from build123d import *

# Parameters (mm, degrees)
CROQUIS1_W              = 36
CROQUIS1_H              = 36
SALIENTE_EXTRUIR1_DEPTH = 13
CROQUIS5_R              = 1.5
CORTAR_EXTRUIR2_DEPTH   = 13
CROQUIS6_W              = 36
CROQUIS6_H              = 36
CROQUIS6_R              = 2.5
CORTAR_EXTRUIR3_DEPTH   = 5
CROQUIS7_W              = 36
CROQUIS7_H              = 36
CROQUIS7_R              = 2.7
CORTAR_EXTRUIR4_DEPTH   = 5
CROQUIS8_W              = 9
CROQUIS8_H              = 10
CROQUIS8_W_2            = 11
CORTAR_EXTRUIR5_DEPTH   = 3


with BuildPart() as part:
    # Croquis1 → Saliente-Extruir1 (new body)
    with BuildSketch(Plane.XY):
        with Locations((-24.893753741, 2.264150943)):
            Rectangle(CROQUIS1_W, CROQUIS1_H)
    extrude(amount=SALIENTE_EXTRUIR1_DEPTH)

    # Croquis5 → Cortar-Extruir2 (cut)
    with BuildSketch(Plane(origin=(0, 0, 0), x_dir=(-1, 0, 0), z_dir=(0, 0, -1))):
        with Locations((40.143753741, 17.514150943)):
            Circle(CROQUIS5_R)
        with Locations((40.143753741, -12.985849057)):
            Circle(CROQUIS5_R)
        with Locations((9.643753741, -12.985849057)):
            Circle(CROQUIS5_R)
        with Locations((9.643753741, 17.514150943)):
            Circle(CROQUIS5_R)
    extrude(amount=-CORTAR_EXTRUIR2_DEPTH, mode=Mode.SUBTRACT)

    # Croquis6 → Cortar-Extruir3 (cut)
    with BuildSketch(Plane(origin=(0, 0, 0), x_dir=(-1, 0, 0), z_dir=(0, 0, -1))):
        with Locations((24.893753741, 2.264150943)):
            Rectangle(CROQUIS6_W, CROQUIS6_H)
        with Locations((40.143753741, 17.514150943)):
            Circle(CROQUIS6_R, mode=Mode.SUBTRACT)
        with Locations((9.643753741, 17.514150943)):
            Circle(CROQUIS6_R, mode=Mode.SUBTRACT)
        with Locations((40.143753741, -12.985849057)):
            Circle(CROQUIS6_R, mode=Mode.SUBTRACT)
        with Locations((9.643753741, -12.985849057)):
            Circle(CROQUIS6_R, mode=Mode.SUBTRACT)
    extrude(amount=-CORTAR_EXTRUIR3_DEPTH, mode=Mode.SUBTRACT)

    # Croquis7 → Cortar-Extruir4 (cut)
    with BuildSketch(Plane.XY.offset(13)):
        with Locations((-24.893753741, 2.264150943)):
            Rectangle(CROQUIS7_W, CROQUIS7_H)
        with Locations((-40.143753741, 17.514150943)):
            Circle(CROQUIS7_R, mode=Mode.SUBTRACT)
        with Locations((-9.643753741, 17.514150943)):
            Circle(CROQUIS7_R, mode=Mode.SUBTRACT)
        with Locations((-40.143753741, -12.985849057)):
            Circle(CROQUIS7_R, mode=Mode.SUBTRACT)
        with Locations((-9.643753741, -12.985849057)):
            Circle(CROQUIS7_R, mode=Mode.SUBTRACT)
    extrude(amount=-CORTAR_EXTRUIR4_DEPTH, mode=Mode.SUBTRACT)

    # Croquis8 → Cortar-Extruir5 (cut)
    with BuildSketch(Plane.XY.offset(8)):
        with Locations((-32.393753741, -4.735849057)):
            Rectangle(CROQUIS8_W, CROQUIS8_H)
        with Locations((-32.393753741, 9.264150943)):
            Rectangle(CROQUIS8_W, CROQUIS8_H)
        with Locations((-18.393753741, -4.735849057)):
            Rectangle(CROQUIS8_W_2, CROQUIS8_H)
        with Locations((-18.393753741, 9.264150943)):
            Rectangle(CROQUIS8_W_2, CROQUIS8_H)
    extrude(amount=-CORTAR_EXTRUIR5_DEPTH, mode=Mode.SUBTRACT)


solid = part.part
Here's how the part is built. I have some questions about the finished solid (model axes, mm). A direction names the side the tool comes from. Coordinates: 2 decimals unless noted, no trailing zeros. Order: outer loops, then holes, each group sorted by start corner. A loop starts at its lowest first (then second) coordinate and runs counter-clockwise, first axis right, second up. Notation, with made-up numbers: M 35.5,38.25 L 93.5,38.25 A28 ccw 93.5,68.25 Z; hole C 84,37.5 d10. An arc over 180 degrees is marked long. Answer as CSV lines item,"result". Start each with the question number.
1. For pin 1 (1.5 mm diameter, centred on y = -10, z = 1.5, fed in from +X); pin 2 (2 mm diameter, centred on x = -35, y = -9, fed in from +Z); pin 3 (18 mm diameter, centred on x = -33.5, y = -4, fed in from -Z), each with a flat end and sliding along its axis, tell me the tip position at first contact or that it passes through.
2. I want a section at A-A, the plane z = 11. Write out the boundary of the cut face in (x, y), and give its area (3 significant figures).
3. I want a section at C-C, the plane y = -8. Write out the boundary of the cut face in (x, z), and give its area (3 significant figures).
4. I need wall thicknesses on line 1 (X direction, y = 7.5, z = 5.25); line 2 (X direction, y = 17.5, z = 3.25); line 3 (X direction, y = 17, z = 5.5). Which ranges of each line are inside material? Lowest first, please. Write a range as [from, to].
5. I want a section at B-B, the plane x = -19. Write out the boundary of the cut face in (y, z).
6. I want a section at D-D, the plane z = 2.5. Write out the boundary of the cut face in (x, y).
7. On a 3-axis mill with a long thin cutter (end or side, diameter ignored), from which of +Z, -Z, +X, -X, +Y, -Y can I reach the whole of each face in a straight line? I mean faces 1 (the cylindrical face through (-9.318, 19.993, 2.465)), 2 (the cylindrical face through (-42.134, 19.339, 10.535)), 3 (the flat face through (-6.894, 2, 6)), 4 (the flat face through (-18, -9.736, 7)). Say none if no direction works.
Recorded:
1,pin 1,"stops at x = -8.53"
1,pin 2,"stops at z = 8"
1,pin 3,"stops at z = 0"
2,outline,"C -40.14,-12.99 d5.4; C -40.14,17.51 d5.4; C -9.64,-12.99 d5.4; C -9.64,17.51 d5.4; hole C -40.14,-12.99 d3; hole C -40.14,17.51 d3; hole C -9.64,-12.99 d3; hole C -9.64,17.51 d3"
2,area,"63.3 mm2"
3,outline,"M -42.89,5 L -36.89,5 L -36.89,8 L -42.89,8 Z; M -27.89,5 L -23.89,5 L -23.89,8 L -27.89,8 Z; M -12.89,5 L -6.89,5 L -6.89,8 L -12.89,8 Z"
3,area,"48.0 mm2"
4,line 1,"x = [-42.89, -36.89], [-27.89, -23.89], [-12.89, -6.89]"
4,line 2,"x = [-42.64, -41.64], [-38.64, -37.64], [-12.14, -11.14], [-8.14, -7.14]"
4,line 3,"x = [-42.89, -41.55], [-38.73, -11.05], [-8.23, -6.89]"
5,outline,"M -15.74,5 L -9.74,5 L -9.74,8 L -15.74,8 Z; M 0.26,5 L 4.26,5 L 4.26,8 L 0.26,8 Z; M 14.26,5 L 20.26,5 L 20.26,8 L 14.26,8 Z"
6,outline,"C -40.14,-12.99 d5; C -40.14,17.51 d5; C -9.64,-12.99 d5; C -9.64,17.51 d5; hole C -40.14,-12.99 d3; hole C -40.14,17.51 d3; hole C -9.64,-12.99 d3; hole C -9.64,17.51 d3"
7,face 1,"-Z"
7,face 2,"+Z"
7,face 3,"+Z, -Z, +X, +Y, -Y"
7,face 4,"+Z, -Z"
